```python
from build123d import *

# Parameters (mm, degrees)
SKETCH_1_R      = 1.6
SKETCH_1_R_2    = 3.1
EXTRUDE_1_DEPTH = 5
FILLET_1_R      = 10


with BuildPart() as part:
    # 草图1 → 凸台-拉伸1 (new body)
    with BuildSketch(Plane.XY):
        Polygon((-7.5, 71), (-7.5, -7.5), (71, -7.5), (71, 37.5), (42.5, 71), align=None)
        Circle(SKETCH_1_R, mode=Mode.SUBTRACT)
        with Locations((0, 15)):
            Circle(SKETCH_1_R, mode=Mode.SUBTRACT)
        with Locations((0, 35)):
            Circle(SKETCH_1_R, mode=Mode.SUBTRACT)
        with Locations((0, 65)):
            Circle(SKETCH_1_R, mode=Mode.SUBTRACT)
        with Locations((15, 0)):
            Circle(SKETCH_1_R, mode=Mode.SUBTRACT)
        with Locations((35, 0)):
            Circle(SKETCH_1_R, mode=Mode.SUBTRACT)
        with Locations((65, 0)):
            Circle(SKETCH_1_R, mode=Mode.SUBTRACT)
        with Locations((16, 58.5)):
            Circle(SKETCH_1_R_2, mode=Mode.SUBTRACT)
        with Locations((16, 13.5)):
            Circle(SKETCH_1_R_2, mode=Mode.SUBTRACT)
        with Locations((46, 13.5)):
            Circle(SKETCH_1_R_2, mode=Mode.SUBTRACT)
        with Locations((46, 58.5)):
            Circle(SKETCH_1_R_2, mode=Mode.SUBTRACT)
    extrude(amount=EXTRUDE_1_DEPTH)

    # 圆角1
    fillet_1_edges = [part.edges().sort_by_distance(p)[0] for p in [
        (42.5, 71, 2.5),
        (71, 37.5, 2.5),
        (71, -7.5, 2.5),
        (-7.5, -7.5, 2.5),
        (-7.5, 71, 2.5),
    ]]
    fillet(fillet_1_edges, radius=FILLET_1_R)


solid = part.part
```
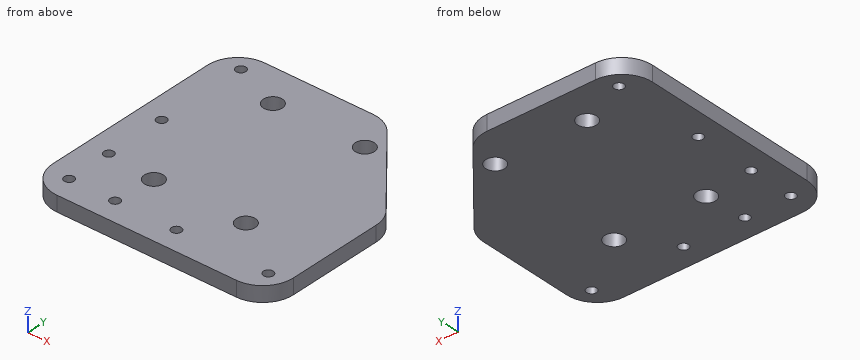
Design review of the part built by this model. Coordinates are the model's own, in mm. Round coordinates to 2 decimals unless told otherwise and drop trailing zeros. Order: outer loops, then holes, each group sorted by start corner. A loop starts at its lowest first (then second) coordinate and runs counter-clockwise, first axis right, second up. Notation, with made-up numbers: (69.5, -24) - (91.5, -24) arc R27 ccw to (91.5, -4) - close; hole circle Ø9 at (66, -38.75). An arc over 180 degrees is marked (long way). Return JSON: item names as keys, results as strings.
Q1. Consider section C-C on x = 35.5. Write out the cut boundary in (y, z).
Computed values:
{"outline": "(-7.5, 0) - (-1.52, 0) - (-1.52, 5) - (-7.5, 5) - close; (1.52, 0) - (71, 0) - (71, 5) - (1.52, 5) - close"}
Q2. Consider section B-B on y = 58.5. Write out the cut boundary in (x, z).
Computed values:
{"outline": "(-7.5, 0) - (12.9, 0) - (12.9, 5) - (-7.5, 5) - close; (19.1, 0) - (42.9, 0) - (42.9, 5) - (19.1, 5) - close; (49.1, 0) - (53.13, 0) - (53.13, 5) - (49.1, 5) - close"}
Q3. For pin 1 Ø3 at (y, z) = (39.5, 4) entering from +X; pin 2 Ø1.5 at (x, z) = (40, 3) entering from +Y, all flat-tipped, find the tip position at first contact; note any pin that passes through.
Computed values:
{"pin 1": "stops at x = 70.09", "pin 2": "stops at y = 70.91"}
Q4. Consider section D-D on y = 15. Write out the cut boundary in (x, z), plus the area to 3 significant figures.
Computed values:
{"outline": "(-7.5, 0) - (-1.6, 0) - (-1.6, 5) - (-7.5, 5) - close; (1.6, 0) - (13.29, 0) - (13.29, 5) - (1.6, 5) - close; (18.71, 0) - (43.29, 0) - (43.29, 5) - (18.71, 5) - close; (48.71, 0) - (71, 0) - (71, 5) - (48.71, 5) - close", "area": "322 mm2"}
Q5. Consider section A-A on z = 0.8. Give the number of separate pieces and of enclosed holes in the cut face, plus the area to 3 significant figures.
Computed values:
{"separate pieces": "1", "enclosed holes": "11", "area": "5,440 mm2"}
Q6. Wall thickness on L1, parallel to Y at x = 0, z = 2.4; L2, parallel to Y at x = 16, z = 3.15; L3, parallel to Y at x = -1, z = 0.95: over which ranges is each line inside the solid? List them lowest first. Write a range as [from, to].
Computed values:
{"L1": "y = [-7.18, -1.6], [1.6, 13.4], [16.6, 33.4], [36.6, 63.4], [66.6, 70.68]", "L2": "y = [-7.5, -1.25], [1.25, 10.4], [16.6, 55.4], [61.6, 71]", "L3": "y = [-6.87, -1.25], [1.25, 13.75], [16.25, 33.75], [36.25, 63.75], [66.25, 70.37]"}
